The model under review builds one solid part; all positions refer to its coordinate system, in mm. A direction names the side the tool comes from. Coordinates: 2 decimals unless noted, no trailing zeros. Write each loop counter-clockwise with the first axis right and the second up, starting at its lowest first coordinate (ties: lowest second). Pieces come first, ordered by that corner, then holes. Notation, with made-up numbers: (-16, -12.5) -> (39, -12.5) arc R24 ccw to (39, 13.5) -> close; hole circle Ø7 at (89, 74). An arc over 180 degrees is marked (long way). Write each question's results on one line, items separated by ' | '.
```python
from build123d import *

# Parameters (mm, degrees)
SKETCH_1_W          = 21
SKETCH_1_H          = 20
SKETCH_1_R          = 5.1
EXTRUDE_1_DEPTH     = 6
FILLET_1_R          = 10
FILLET_2_R          = 2
SKETCH_2_W          = 7
SKETCH_2_H          = 6
EXTRUDE_2_DEPTH     = 6
SKETCH_3_R          = 1
CUT_EXTRUDE_1_DEPTH = 10


with BuildPart() as part:
    # 스케치1 → 보스-돌출1 (new body)
    with BuildSketch(Plane(origin=(0, 0, 0), x_dir=(0, 0, -1), z_dir=(1, 0, 0))):
        with Locations((10.5, 10)):
            Rectangle(SKETCH_1_W, SKETCH_1_H)
        with Locations((8, 10)):
            Circle(SKETCH_1_R, mode=Mode.SUBTRACT)
    extrude(amount=EXTRUDE_1_DEPTH)

    # 필렛1
    fillet_1_edges = [part.edges().sort_by_distance(p)[0] for p in [
        (3, 20, -21),
    ]]
    fillet(fillet_1_edges, radius=FILLET_1_R)

    # 필렛2
    fillet_2_edges = [part.edges().sort_by_distance(p)[0] for p in [
        (3, 20, 0),
    ]]
    fillet(fillet_2_edges, radius=FILLET_2_R)

    # 스케치2 → 보스-돌출2 (add)
    with BuildSketch(Plane(origin=(6, 0, 0), x_dir=(0, 0, -1), z_dir=(1, 0, 0))):
        with Locations((10.5, -3)):
            Rectangle(SKETCH_2_W, SKETCH_2_H)
    extrude(amount=-EXTRUDE_2_DEPTH)

    # 스케치3 → 컷-돌출1 (cut)
    with BuildSketch(Plane(origin=(6, 0, 0), x_dir=(0, 0, -1), z_dir=(1, 0, 0))):
        with Locations((15, 0)):
            Circle(SKETCH_3_R)
        with Locations((6, 0)):
            Circle(SKETCH_3_R)
    extrude(amount=-CUT_EXTRUDE_1_DEPTH, mode=Mode.SUBTRACT)


solid = part.part
```
Q1. For line 1 (Y direction, x = 1.75, z = -8); line 2 (Y direction, x = 5.1, z = -2.25); line 3 (Y direction, x = 1.25, z = -9.25), list the stretches that pass through material, from the lowest coordinate up. Write a range as from..to.
Solution:
line 1: -6..4.9, 15.1..20 | line 2: 0..20 | line 3: -6..5.06, 14.94..20
Q2. Add section D-D (z = -2.5). Write out the cut boundary in (x, y), plus the area to 3 significant figures.
Solution:
outline: (0, 0) -> (6, 0) -> (6, 20) -> (0, 20) -> close | area: 120 mm²
Q3. Add section B-B (y = 8.5). Write out the cut boundary in (x, z), plus the area to 3 significant figures.
Solution:
outline: (0, -21) -> (6, -21) -> (6, -12.87) -> (0, -12.87) -> close; (0, -3.13) -> (6, -3.13) -> (6, 0) -> (0, 0) -> close | area: 67.5 mm²
Q4. Machinability: for faces 1 (the flat face through (3, 0, -2)), 2 (the flat face through (3, -3, -14)), 3 (the flat face through (3, 20, -6)), which of the approach directions +Z, -Z, +X, -X, +Y, -Y give a long, thin tool a straight path to every point of the face, cutting with its end or side? Answer none if there is none.
Solution:
face 1: +Z, +X, -X, -Y | face 2: -Z, +X, -X, -Y | face 3: +Z, -Z, +X, -X, +Y
Q5. Clearance check with flat-ended pins moving along their axes: P1, Ø3, axis at x = 2.5, z = -2.5, coming from the -Y side; P2, Ø3, axis at x = 4, y = -3, coming from the -Z side. State where each tip first meets the part, or that it passes through.
Solution:
P1: y = 0 | P2: z = -14
Q6. Add section C-C (x = 3.4). Write out the cut boundary in (y, z), plus the area to 3 significant figures.
Solution:
outline: (-6, -14) -> (0, -14) arc R1 cw to (0, -16) -> (0, -21) -> (10, -21) arc R10 ccw to (20, -11) -> (20, -2) arc R2 ccw to (18, 0) -> (0, 0) -> (0, -5) arc R1 cw to (0, -7) -> (-6, -7) -> close; hole circle Ø10.2 at (10, -8) | area: 355 mm²
Q7. Add section A-A (z = -6.25). Write out the cut boundary in (x, y), plus the area to 3 significant figures.
Solution:
outline: (0, 0.97) -> (6, 0.97) -> (6, 5.21) -> (0, 5.21) -> close; (0, 14.79) -> (6, 14.79) -> (6, 20) -> (0, 20) -> close | area: 56.7 mm²
